```python
from build123d import *

# Parameters (mm, degrees)
SKETCH1_R           = 20
SKETCH1_R_2         = 6.35
BOSS_EXTRUDE1_DEPTH = 3
SKETCH2_R           = 5
BOSS_EXTRUDE2_DEPTH = 3
FILLET1_R           = 10
FILLET2_R           = 10
FILLET3_R           = 3
FILLET4_R           = 3


with BuildPart() as part:
    # Sketch1 → Boss-Extrude1 (new body)
    # profile 1 of 2: a face of its own
    with BuildSketch(Plane(origin=(0, 0, 0), x_dir=(1, 0, 0), z_dir=(0, 1, 0))):
        with BuildLine():
            Line((-20, 50), (-20, 0))
            ThreePointArc((-20, 0), (0, 20), (20, 0))
            Line((20, 0), (20, 50))
            Line((20, 50), (-20, 50))
        make_face()
    # profile 2 of 2: a face of its own
    with BuildSketch(Plane(origin=(0, 0, 0), x_dir=(1, 0, 0), z_dir=(0, 1, 0))):
        Circle(SKETCH1_R)
        with Locations(Location((0, 0, 0), (0, 0, 270))):
            Circle(SKETCH1_R_2, mode=Mode.SUBTRACT)
    extrude(amount=BOSS_EXTRUDE1_DEPTH)

    # Sketch2 → Boss-Extrude2 (add)
    with BuildSketch(Plane(origin=(0, 0, -50), x_dir=(-1, 0, 0), z_dir=(0, 0, -1))):
        with BuildLine():
            Line((-20, 3), (-20, 50))
            ThreePointArc((-20, 50), (0, 70), (20, 50))
            Line((20, 50), (20, 3))
            Line((20, 3), (20, 0))
            Line((20, 0), (-20, 0))
            Line((-20, 0), (-20, 3))
        make_face()
        with Locations((0, 50)):
            Circle(SKETCH2_R, mode=Mode.SUBTRACT)
    extrude(amount=-BOSS_EXTRUDE2_DEPTH)

    # Fillet1
    fillet1_edges = [part.edges().sort_by_distance(p)[0] for p in [
        (0, 3, -47),
    ]]
    fillet(fillet1_edges, radius=FILLET1_R)

    # Fillet2
    fillet2_edges = [part.edges().sort_by_distance(p)[0] for p in [
        (0, 0, -50),
    ]]
    fillet(fillet2_edges, radius=FILLET2_R)

    # Fillet3
    fillet3_edges = [part.edges().sort_by_distance(p)[0] for p in [
        (20, 5.928932188, -44.071067812),
        (20, 31.5, -47),
        (0, 70, -47),
        (-20, 31.5, -47),
        (-20, 5.928932188, -44.071067812),
        (0, 3, -6.35),
        (0, 3, 20),
        (-20, 3, -18.5),
        (20, 3, -18.5),
    ]]
    fillet(fillet3_edges, radius=FILLET3_R - 0.0001)  # a hair under: the kernel refuses the full size

    # Fillet4
    fillet4_edges = [part.edges().sort_by_distance(p)[0] for p in [
        (5, 50, -47),
    ]]
    fillet(fillet4_edges, radius=FILLET4_R - 0.0001)  # a hair under: the kernel refuses the full size


solid = part.part
```
The model under review builds one solid part; all positions refer to its coordinate system, in mm. A direction names the side the tool comes from. Round coordinates to 2 decimals unless told otherwise and drop trailing zeros. Answer as a JSON object with one key per item and string values. Group by question number.
1) We need section A-A on x = 0. Give the number of separate pieces and of enclosed holes in the cut face, then the cut area to 3 significant figures.
2) For faces 1 (the face through (0, 3, -16)), 2 (the face through (19.14, 2.1, -18.24)), 3 (the face through (0, 0, -10)), 4 (the face through (0, 40, -50)), 5 (the face through (-19.14, 31.76, -47.9)), list the 3-axis set-ups (+Z, -Z, +X, -X, +Y, -Y) from which the entire face can be reached by the end or side of a thin tool; tool diameter is ignored.
3) For pin 1 Ø4 at (x, y) = (-1.5, 21) entering from +Z; pin 2 Ø10 at (x, z) = (2.5, -8.5) entering from +Y; pin 3 Ø9 at (x, y) = (0, 50) entering from +Z, all flat-tipped, find the tip position at first contact; note any pin that passes through.
4) For line 1 (Z direction, x = 15.5, y = 33); line 2 (Y direction, x = 10.5, z = 1.5); line 3 (X direction, y = 50, z = -49.95), list the stretches that pass through material, from the lowest coordinate up. Write a range as [from, to].
Result set:
{
 "1": {"separate pieces": "3", "enclosed holes": "0", "area": "331 mm²"},
 "2": {"face 1": "+Z, +X, -X, +Y", "face 2": "+Z, +X, +Y", "face 3": "+Z, -Z, +X, -X, -Y", "face 4": "-Z, +X, -X, +Y, -Y", "face 5": "+Z, -X, +Y"},
 "3": {"pin 1": "z = -47", "pin 2": "y = 3", "pin 3": "through"},
 "4": {"line 1": "[-50, -47]", "line 2": "[0, 3]", "line 3": "[-20, -5], [5, 20]"}
}
